Can you work these out from the model? Positions are in its coordinate system, mm. A direction names the side the tool comes from. Give positions to 0.01 mm unless a question says otherwise; leave off trailing zeros. Order: outer loops, then holes, each group sorted by start corner. A loop starts at its lowest first (then second) coordinate and runs counter-clockwise, first axis right, second up. Notation, with made-up numbers: M 85,81.25 L 120,81.25 A26 ccw 120,102.25 Z; hole C -9,47 d5. An arc over 180 degrees is marked long. Answer as a JSON object with one key per item and string values.
```python
from build123d import *

# Parameters (mm, degrees)
BOSS_EXTRUDE1_DEPTH = 10
SKETCH2_R           = 1.5
CUT_EXTRUDE1_DEPTH  = 141.05802369
CUT_EXTRUDE2_REACH  = 142.058
SKETCH3_R           = 1.5
CHAMFER2_SIZE       = 7
CUT_EXTRUDE3_REACH  = 124.28
CUT_EXTRUDE4_REACH  = 136.001
SKETCH5_R           = 1.5
SKETCH9_R           = 3.5
CUT_EXTRUDE7_DEPTH  = 3
CUT_EXTRUDE8_START  = -3
SKETCH10_R          = 3.5
CUT_EXTRUDE8_DEPTH  = 3


with BuildPart() as part:
    # Sketch1 → Boss-Extrude1 (new body)
    with BuildSketch(Plane(origin=(0, 0, 0), x_dir=(-1, 0, 0), z_dir=(0, 0, 1))):
        Polygon((47.5, 36.642135619), (47.5, 56.593701556), (55.5, 56.593701556), (55.5, 30.499999996), (55.5, 21.076918494), (25, 0), (0, 0), (-32.5, 27.270738013), (-32.5, 40.5), (-32.5, 108.5), (-7.5, 108.5), (-7.5, 98.5), (-22.5, 98.5), (-22.5, 32.416456895), (-13.661410851, 25), (35.857864376, 25), (43.690340999, 25), (47.5, 27.632651549), align=None)
    extrude(amount=BOSS_EXTRUDE1_DEPTH)

    # Sketch2 → Cut-Extrude1 (cut, through all)
    with BuildSketch(Plane.ZY.offset(55.5)):
        with Locations(Location((5, -51.593701556, 0), (0, 0, 270))):
            Circle(SKETCH2_R)
    extrude(amount=-CUT_EXTRUDE1_DEPTH, mode=Mode.SUBTRACT)

    # Sketch3 → Cut-Extrude2 (cut, up to next)
    with BuildSketch(Plane(origin=(32.5, 0, 0), x_dir=(0, 0, -1), z_dir=(1, 0, 0)), mode=Mode.PRIVATE) as cut_extrude2_sk1:
        with Locations(Location((-5, -77.593701556, 0), (0, 0, 90))):
            Circle(SKETCH3_R)
    cut_extrude2_tool1 = extrude(cut_extrude2_sk1.sketch, amount=-CUT_EXTRUDE2_REACH, mode=Mode.PRIVATE) & part.part
    add(cut_extrude2_tool1.solids().sort_by_distance((32.5, -77.593702, 5))[0], mode=Mode.SUBTRACT)

    # Chamfer2
    chamfer2_edges = [part.edges().sort_by_distance(p)[0] for p in [
        (22.5, -98.5, 5),
    ]]
    chamfer(chamfer2_edges, length=CHAMFER2_SIZE)

    # Sketch4 → Cut-Extrude3 (cut, up to next)
    with BuildSketch(Plane.XY.offset(10), mode=Mode.PRIVATE) as cut_extrude3_sk1:
        Polygon((22.5, -108.5), (22.5, -101.5), (32.5, -91.5), (32.5, -108.5), align=None)
    cut_extrude3_tool1 = extrude(cut_extrude3_sk1.sketch, amount=-CUT_EXTRUDE3_REACH, mode=Mode.PRIVATE) & part.part
    add(cut_extrude3_tool1.solids().sort_by_distance((28.194444, -102.152778, 10))[0], mode=Mode.SUBTRACT)

    # Sketch5 → Cut-Extrude4 (cut, up to next)
    with BuildSketch(Plane(origin=(22.5, 0, 0), x_dir=(0, 0, -1), z_dir=(1, 0, 0)), mode=Mode.PRIVATE) as cut_extrude4_sk1:
        with Locations((-5, -104.593701556)):
            Circle(SKETCH5_R)
    cut_extrude4_tool1 = extrude(cut_extrude4_sk1.sketch, amount=-CUT_EXTRUDE4_REACH, mode=Mode.PRIVATE) & part.part
    add(cut_extrude4_tool1.solids().sort_by_distance((22.5, -104.593702, 5))[0], mode=Mode.SUBTRACT)

    # Sketch9 → Cut-Extrude7 (cut)
    with BuildSketch(Plane(origin=(-47.5, 0, 0), x_dir=(0, 0, -1), z_dir=(1, 0, 0))):
        with Locations((-1.036207833, -38.166551759)):
            Circle(SKETCH9_R)
    extrude(amount=-CUT_EXTRUDE7_DEPTH, mode=Mode.SUBTRACT)

    # Sketch10 → Cut-Extrude8 (cut)
    with BuildSketch(Plane.ZY.offset(-22.5).offset(CUT_EXTRUDE8_START)):
        with Locations((1.036207833, -38.166551759)):
            Circle(SKETCH10_R)
        with Locations((1.036207833, -64.166551759)):
            Circle(SKETCH10_R)
    extrude(amount=CUT_EXTRUDE8_DEPTH, mode=Mode.SUBTRACT)


solid = part.part
```
1) I want a section at C-C on y = -62.5. Write out the boundary of the cut face in (x, z), and give its area (3 significant figures).
Results found:
{"outline": "M 22.5,4.11 L 25.5,4.11 L 25.5,0 L 32.5,0 L 32.5,10 L 22.5,10 Z", "area": "87.7 mm²"}
2) I want a section at B-B on x = -12. Write out the boundary of the cut face in (y, z), and give its area (3 significant figures).
Results found:
{"outline": "M -25,0 L 0,0 L 0,10 L -25,10 Z", "area": "250 mm²"}
3) I'm going to push flat-ended pins straight in: pin 1 Ø5 at (y, z) = (-63, 2) entering from -X; pin 2 Ø3.5 at (y, z) = (-104, 7.5) entering from +X; pin 3 Ø2.5 at (y, z) = (-77.59, 5) entering from +X; pin 4 Ø4 at (y, z) = (-64.17, 1.04) entering from -X. Where does each tip first touch, or does it pass through?
Results found:
{"pin 1": "stops at x = 22.5", "pin 2": "stops at x = 22.5", "pin 3": "passes through", "pin 4": "stops at x = 25.5"}
4) For faces 1 (the face through (-51, -56.594, 5)), 2 (the face through (-47.5, -42, 5)), 3 (the face through (18.14, -28.76, 4.93)), which set-ups out of +Z, -Z, +X, -X, +Y, -Y let a thin tool reach every point of the face, with its end or its side?
Results found:
{"face 1": "+Z, -Z, -X, -Y", "face 2": "+Z, -Z, -Y", "face 3": "+Z, -Z"}
5) I need wall thicknesses on L1, parallel to Y at x = 29.5, z = 4.75; L2, parallel to Y at x = -21, z = 8.25; L3, parallel to X at y = -77, z = 2. Which ranges of each line are inside material? Lowest first, please.
Results found:
{"L1": "y = -94.5 to -79.07, -76.11 to -53.07, -50.11 to -24.75", "L2": "y = -25 to 0", "L3": "x = 22.5 to 32.5"}
6) Thinking about a two-plate mould opening in Z: for faces 4 (the face through (11, -98.5, 5)), 5 (the face through (-8, -22, 0)), 6 (the face through (-51.56, -50.4, 4.09)), which applies, pulls with the +Z half, pulls with the -Z half, needs draft (parallel to the pull), parting line crosses it, or undercut?
Results found:
{"face 4": "needs draft", "face 5": "pulls with the -Z half", "face 6": "undercut"}
7) I want a section at A-A on z = 7.75. Write out the boundary of the cut face in (x, y).
Results found:
{"outline": "M -55.5,-56.59 L -47.5,-56.59 L -47.5,-27.63 L -43.69,-25 L 13.66,-25 L 22.5,-32.42 L 22.5,-91.5 L 15.5,-98.5 L 7.5,-98.5 L 7.5,-108.5 L 22.5,-108.5 L 22.5,-101.5 L 32.5,-91.5 L 32.5,-27.27 L 0,0 L -25,0 L -55.5,-21.08 Z"}
